from build123d import *

# Parameters (mm, degrees)
BOSS_EXTRUDE1_DEPTH = 1.5
BOSS_EXTRUDE2_DEPTH = 2


with BuildPart() as part:
    # Sketch1 → Boss-Extrude1 (new body)
    with BuildSketch(Plane.XY):
        with BuildLine():
            Line((19.723160965, -30.122), (15.214660965, -41.425))
            Line((15.214660965, -41.425), (15.214660965, -45.122))
            Line((15.214660965, -45.122), (35.1855, -45.122))
            ThreePointArc((35.1855, -45.122), (42.256567812, -42.193067812), (45.1855, -35.122))
            Line((45.1855, -35.122), (45.1855, -30.122))
            Line((45.1855, -30.122), (45.1855, 35.122))
            ThreePointArc((45.1855, 35.122), (42.256567812, 42.193067812), (35.1855, 45.122))
            Line((35.1855, 45.122), (-35.1855, 45.122))
            ThreePointArc((-35.1855, 45.122), (-42.256567812, 42.193067812), (-45.1855, 35.122))
            Line((-45.1855, 35.122), (-45.1855, -30.122))
            Line((-45.1855, -30.122), (-45.1855, -35.122))
            ThreePointArc((-45.1855, -35.122), (-42.256567812, -42.193067812), (-35.1855, -45.122))
            Line((-35.1855, -45.122), (-15.086607553, -45.122))
            Line((-15.086607553, -45.122), (-15.086607553, -41.425))
            Line((-15.086607553, -41.425), (-19.722107553, -30.122))
            Line((-19.722107553, -30.122), (-24.9555, -30.122))
            ThreePointArc((-24.9555, -30.122), (-28.653668466, -28.590168466), (-30.1855, -24.892))
            Line((-30.1855, -24.892), (-30.1855, 24.892))
            ThreePointArc((-30.1855, 24.892), (-28.653668466, 28.590168466), (-24.9555, 30.122))
            Line((-24.9555, 30.122), (24.9555, 30.122))
            ThreePointArc((24.9555, 30.122), (28.653668466, 28.590168466), (30.1855, 24.892))
            Line((30.1855, 24.892), (30.1855, -24.892))
            ThreePointArc((30.1855, -24.892), (28.653668466, -28.590168466), (24.9555, -30.122))
            Line((24.9555, -30.122), (19.723160965, -30.122))
        make_face()
    extrude(amount=-BOSS_EXTRUDE1_DEPTH)

    # Sketch2 → Boss-Extrude2 (add)
    with BuildSketch(Plane.XY):
        with BuildLine():
            Line((-24.9555, 30.122), (24.9555, 30.122))
            ThreePointArc((24.9555, 30.122), (28.653668466, 28.590168466), (30.1855, 24.892))
            Line((30.1855, 24.892), (30.1855, -24.892))
            ThreePointArc((30.1855, -24.892), (28.653668466, -28.590168466), (24.9555, -30.122))
            Line((24.9555, -30.122), (19.723160965, -30.122))
            Line((19.723160965, -30.122), (15.214660965, -41.425))
            Line((15.214660965, -41.425), (15.214660965, -45.122))
            Line((15.214660965, -45.122), (35.1855, -45.122))
            ThreePointArc((35.1855, -45.122), (42.256567812, -42.193067812), (45.1855, -35.122))
            Line((45.1855, -35.122), (45.1855, 35.122))
            ThreePointArc((45.1855, 35.122), (42.256567812, 42.193067812), (35.1855, 45.122))
            Line((35.1855, 45.122), (-35.1855, 45.122))
            ThreePointArc((-35.1855, 45.122), (-42.256567812, 42.193067812), (-45.1855, 35.122))
            Line((-45.1855, 35.122), (-45.1855, -35.122))
            ThreePointArc((-45.1855, -35.122), (-42.256567812, -42.193067812), (-35.1855, -45.122))
            Line((-35.1855, -45.122), (-15.086607553, -45.122))
            Line((-15.086607553, -45.122), (-15.086607553, -41.425))
            Line((-15.086607553, -41.425), (-19.722107553, -30.122))
            Line((-19.722107553, -30.122), (-24.9555, -30.122))
            ThreePointArc((-24.9555, -30.122), (-28.653668466, -28.590168466), (-30.1855, -24.892))
            Line((-30.1855, -24.892), (-30.1855, 24.892))
            ThreePointArc((-30.1855, 24.892), (-28.653668466, 28.590168466), (-24.9555, 30.122))
        make_face()
        with BuildLine():
            Line((-19.722107553, -30.122), (-15.086607553, -41.425))
            Line((-15.086607553, -41.425), (-15.086607553, -36.275))
            Line((-15.086607553, -36.275), (15.214660965, -36.275))
            Line((15.214660965, -36.275), (15.214660965, -41.425))
            Line((15.214660965, -41.425), (19.723160965, -30.122))
            Line((19.723160965, -30.122), (24.9555, -30.122))
            ThreePointArc((24.9555, -30.122), (28.653668466, -28.590168466), (30.1855, -24.892))
            Line((30.1855, -24.892), (30.1855, 24.892))
            ThreePointArc((30.1855, 24.892), (28.653668466, 28.590168466), (24.9555, 30.122))
            Line((24.9555, 30.122), (-24.9555, 30.122))
            ThreePointArc((-24.9555, 30.122), (-28.653668466, 28.590168466), (-30.1855, 24.892))
            Line((-30.1855, 24.892), (-30.1855, -24.892))
            ThreePointArc((-30.1855, -24.892), (-28.653668466, -28.590168466), (-24.9555, -30.122))
            Line((-24.9555, -30.122), (-19.722107553, -30.122))
        make_face()
    extrude(amount=BOSS_EXTRUDE2_DEPTH)


solid = part.part
The model under review builds one solid part; all positions refer to its coordinate system, in mm. A direction names the side the tool comes from. Round coordinates to 2 decimals unless told otherwise and drop trailing zeros. Loops run counter-clockwise (first coordinate to the right, second up) from the corner with the lowest first, then second, coordinate; pieces in that order, holes last. Notation, with made-up numbers: M 85,-13.75 L 92,-13.75 A21 ccw 92,6.25 Z; hole C -9,79 d9. An arc over 180 degrees is marked long. Answer as a JSON object with one key per item and string values.
Item 1: We need section B-B, the plane y = -37.5. State the section outline as (x, z) points.
Check sheet entries:
{"outline": "M -44.9,-1.5 L -16.7,-1.5 L -16.7,0 L -15.09,0 L -15.09,2 L -44.9,2 Z; M 15.21,0 L 16.78,0 L 16.78,-1.5 L 44.9,-1.5 L 44.9,2 L 15.21,2 Z"}
Item 2: We need section A-A, the plane z = -0.9. State the section outline as (x, y) points (1 decimal).
Check sheet entries:
{"outline": "M -45.2,-35.1 A10 ccw -35.2,-45.1 L -15.1,-45.1 L -15.1,-41.4 L -19.7,-30.1 L -25,-30.1 A5.2 cw -30.2,-24.9 L -30.2,24.9 A5.2 cw -25,30.1 L 25,30.1 A5.2 cw 30.2,24.9 L 30.2,-24.9 A5.2 cw 25,-30.1 L 19.7,-30.1 L 15.2,-41.4 L 15.2,-45.1 L 35.2,-45.1 A10 ccw 45.2,-35.1 L 45.2,35.1 A10 ccw 35.2,45.1 L -35.2,45.1 A10 ccw -45.2,35.1 Z"}
Item 3: Clearance check with flat-ended pins moving along their axes: P1, Ø2, axis at x = 0.5, z = 0.5, coming from the -Y side (3 decimals); P2, Ø8, axis at x = -6.5, y = -14.5, coming from the -Z side; P3, Ø1.8, axis at y = -41, z = 1, coming from the -X side. State where each tip first meets the part, or that it passes through.
Check sheet entries:
{"P1": "y = -36.275", "P2": "z = 0", "P3": "x = -43.86"}
Item 4: Tool access review of faces 1 (the face through (25, -45.122, 0)), 2 (the face through (28.613, 28.631, -0.74)), 3 (the face through (-15.087, -42, 1)): name each direction out of +Z, -Z, +X, -X, +Y, -Y from which nothing blocks a thin tool from reaching the whole face with its end or side.
Check sheet entries:
{"face 1": "+Z, -Z, +X, -X, -Y", "face 2": "-Z", "face 3": "+Z, -Z, -Y"}
Item 5: We need section C-C, the plane y = -8.5. State the section outline as (x, z) points.
Check sheet entries:
{"outline": "M -45.19,-1.5 L -30.19,-1.5 L -30.19,0 L 30.19,0 L 30.19,-1.5 L 45.19,-1.5 L 45.19,2 L -45.19,2 Z"}
Item 6: We need section D-D, the plane x = 4.5. State the section outline as (y, z) points (3 decimals).
Check sheet entries:
{"outline": "M -36.275,0 L 30.122,0 L 30.122,-1.5 L 45.122,-1.5 L 45.122,2 L -36.275,2 Z"}
Item 7: The part is to be moulded in two halves that separate along Y. For faces 4 (the face through (-1, 31, -1.5)), 5 (the face through (17.5, -35.7, -0.7)), 6 (the face through (0, 45.122, 0)), 7 (the face through (0, -36.275, 1)), say which applies: +Y half, -Y half, draft (parallel to the pull), parting line (faces both ways), or undercut.
Check sheet entries:
{"face 4": "draft", "face 5": "undercut", "face 6": "+Y half", "face 7": "-Y half"}
Item 8: For line 1 along X through (y, z) = (-7, -1.15); line 2 along Y through (x, z) = (20, -0.9); line 3 along Y through (x, z) = (8.5, 1.95) (3 decimals), list the stretches that pass through material, from the lowest coordinate up.
Check sheet entries:
{"line 1": "-45.19 to -30.19, 30.19 to 45.19", "line 2": "-45.12 to -30.12, 30.12 to 45.12", "line 3": "-36.275 to 45.122"}
